Read the model definition and answer for the solid it produces. Units are mm, in the model's axes. A direction names the side the tool comes from. Round coordinates to 2 decimals unless told otherwise and drop trailing zeros. Loops run counter-clockwise (first coordinate to the right, second up) from the corner with the lowest first, then second, coordinate; pieces in that order, holes last. Notation, with made-up numbers: M 9,74 L 37,74 A32 cw 37,100 Z; hole C -12,-2.75 d8. An arc over 180 degrees is marked long. Write each question's results on one line, items separated by ' | '.
Autodesk Inventor part; units mm, degrees
ref_plane "YZ Plane" through (0, 0, 0) normal (1, 0, 0) x (0, 1, 0)
ref_plane "XZ Plane" through (0, 0, 0) normal (0, 1, 0) x (-1, 0, 0)
ref_plane "XY Plane" through (0, 0, 0) normal (0, 0, 1) x (1, 0, 0)
sketch "Szkic1" plane through (0, 0, 0) normal (0, 0, 1) x (1, 0, 0)
  line L0 (-30, -30) -> (30, -30)
  line L1 (30, -30) -> (30, 30)
  line L2 (30, 30) -> (-30, 30)
  line L3 (-30, 30) -> (-30, -30)
  line L4 (-30, -30) -> (30, 30) construction
  line L5 (30, -30) -> (-30, 30) construction
  point P0 (0, 0)
  dimension "d0" = 60
  dimension "d1" = 60
extrude "Wyciągnięcie proste1" add sketch "Szkic1" along normal blind 35
sketch "Szkic2" plane through (0, 0, 35) normal (0, 0, 1) x (1, 0, 0)
  circle A0 centre (0, 0) radius 25
  dimension "d4" = 50
extrude "Wyciągnięcie proste2" cut sketch "Szkic2" against normal blind 12
sketch "Szkic3" plane through (0, 0, 23) normal (0, 0, 1) x (1, 0, 0)
  circle A0 centre (0, 0) radius 14
  dimension "d7" = 28
extrude "Wyciągnięcie proste3" cut sketch "Szkic3" against normal up to next
sketch "Szkic4" plane through (0, 0, 23) normal (0, 0, 1) x (1, 0, 0)
  circle A0 centre (0, 0) radius 19
  circle A1 centre (0, 19) radius 3
  circle A2 centre (-16.4545, 9.5) radius 3
  circle A3 centre (-16.4545, -9.5) radius 3
  circle A4 centre (0, -19) radius 3
  circle A5 centre (16.4545, -9.5) radius 3
  circle A6 centre (16.4545, 9.5) radius 3
  dimension "d10" = 38
  dimension "d11" = 6
  dimension "d14" = 360
sketch "Szkic13" plane through (0, 0, 35) normal (0, 0, 1) x (1, 0, 0)
  circle A0 centre (0, 0) radius 25
  line L0 (-30, -30) -> (30, -30)
  line L1 (30, -30) -> (30, 30)
  line L2 (30, 30) -> (-30, 30)
  line L3 (-30, 30) -> (-30, -30)
extrude "Wyciągnięcie proste10" cut sketch "Szkic13" against normal up to surface (12 mm away)
extrude "Wyciągnięcie proste11" cut sketch "Szkic4" against normal up to next contours A6 A0 | A0 A6 | A5 A0 | A0 A5 | A1 A0 | A0 A1 | A4 A0 | A0 A4 | A2 A0 | A0 A2 | A3 A0 | A0 A3
thread "Gwint7"
thread "Gwint8"
thread "Gwint9"
thread "Gwint10"
thread "Gwint11"
thread "Gwint12"
sketch "Szkic14" plane through (0, 0, 0) normal (0, 0, -1) x (-1, 0, 0)
  circle A0 centre (0, 0) radius 14
  line L0 (30, -30) -> (-30, -30)
  line L1 (30, 30) -> (30, -30)
  line L2 (-30, 30) -> (30, 30)
  line L3 (-30, -30) -> (-30, 30)
extrude "Wyciągnięcie proste12" cut sketch "Szkic14" against normal blind 3
sketch "Szkic16" plane through (-30, -30, 23) normal (0, -1, 0) x (1, 0, 0)
  line L0 (0, -20) -> (60, -20)
  line L1 (60, -20) -> (60, 0)
  line L2 (60, 0) -> (0, 0)
  line L3 (0, -20) -> (0, 0)
  point P0 (30, -23)
extrude "Wyciągnięcie proste14" add sketch "Szkic16" along normal blind 20
sketch "Szkic17" plane through (0, 0, 23) normal (0, 0, 1) x (1, 0, 0)
  circle A0 centre (16.4545, 9.5) radius 3
  circle A1 centre (0, -19) radius 3
  circle A2 centre (-16.4545, 9.5) radius 3
  circle A3 centre (0, 19) radius 3
  circle A4 centre (-16.4545, -9.5) radius 3
  circle A5 centre (16.4545, -9.5) radius 3
  line L0 (30, 30) -> (30, -50)
  line L1 (-30, 30) -> (30, 30)
  line L2 (-30, -50) -> (-30, 30)
  line L3 (30, -50) -> (-30, -50)
  circle A6 centre (0, 0) radius 14
  line L4 (-30, -50) -> (-30, -40)
  line L5 (-30, 30) -> (-30, -50)
  line L6 (-30, -40) -> (30, -40)
  line L7 (30, -50) -> (30, 30)
  line L8 (-30, -40) -> (-18, -40)
  line L9 (-18, -40) -> (-6, -40)
  line L10 (-6, -40) -> (6, -40)
  line L11 (6, -40) -> (18, -40)
  circle A7 centre (-18, -40) radius 2.5
  circle A8 centre (-6, -40) radius 2.5
  circle A9 centre (6, -40) radius 2.5
  circle A10 centre (18, -40) radius 2.5
  dimension "d100" = 10
  dimension "d101" = 12
  dimension "d102" = 12
  dimension "d103" = 12
  dimension "d104" = 12
  dimension "d105" = 5
  dimension "d106" = 5
  dimension "d107" = 5
  dimension "d108" = 5
hole "Otwór1" at (-18, -40, 23) at (-6, -40, 23) at (6, -40, 23) at (18, -40, 23) direction (0, 0, -1) diameter 5 end through all counterbore diameter 9 counterbore depth 5
properties part number "Obudowa nakrętki trapezowej fi 16 - oś Y"
1. Find section B-B, the plane z = 6. Count the separate pieces of the cut face and the enclosed holes in it, then the cut area to 3 significant figures.
Completed:
separate pieces: 1 | enclosed holes: 11 | area: 3,940 mm2
2. Find section A-A, the plane y = 0. Give the vertices of the cut face in (x, z), then the cut area to 3 significant figures.
Completed:
outline: M -30,3 L -14,3 L -14,23 L -30,23 Z; M 14,3 L 30,3 L 30,23 L 14,23 Z | area: 640 mm2
3. Given P1, Ø4, axis at x = -6, y = -40, coming from the +Z side; P2, Ø4.5, axis at x = -7, y = -39, coming from the +Z side, each flat-ended and moving along its own axis, determine where each tip first touches the part or whether it passes through.
Completed:
P1: passes through | P2: stops at z = 18
4. Find section D-D, the plane y = 9.5. Give the vertices of the cut face in (x, z), then the cut area to 3 significant figures.
Completed:
outline: M -30,3 L -19.45,3 L -19.45,23 L -30,23 Z; M -13.45,3 L -10.28,3 L -10.28,23 L -13.45,23 Z; M 10.28,3 L 13.45,3 L 13.45,23 L 10.28,23 Z; M 19.45,3 L 30,3 L 30,23 L 19.45,23 Z | area: 549 mm2
5. Determine the mould class of faces 1 (the face through (-30, -9, 13)), 2 (the face through (19.226, 8.351, 13.14)), 3 (the face through (0, -50, 13)) for opening direction Y: released by +Y, released by -Y, zero draft, split by the parting line, or undercut.
Completed:
face 1: zero draft | face 2: undercut | face 3: released by -Y
6. Find section C-C, the plane x = -6. Give the vertices of the cut face in (y, z).
Completed:
outline: M -50,3 L -42.5,3 L -42.5,18 L -44.5,18 L -44.5,23 L -50,23 Z; M -37.5,3 L -12.65,3 L -12.65,23 L -35.5,23 L -35.5,18 L -37.5,18 Z; M 12.65,3 L 30,3 L 30,23 L 12.65,23 Z
7. Which of the six approach directions +Z, -Z, +X, -X, +Y, -Y give full straight-line access (tool end or side, diameter ignored) to faces 4 (the face through (-19.45, 9.63, 13.14)), 5 (the face through (-7.352, -44.292, 20.465))?
Completed:
face 4: +Z, -Z | face 5: +Z
8. Find the intervals of material crossed by L1, parallel to X at y = -40, z = 22; L2, parallel to X at y = 19, z = 18.5; L3, parallel to X at y = -40, z = 7.25, in increasing order.
Completed:
L1: x = -30 to -22.5, -13.5 to -10.5, -1.5 to 1.5, 10.5 to 13.5, 22.5 to 30 | L2: x = -30 to -3, 3 to 30 | L3: x = -30 to -20.5, -15.5 to -8.5, -3.5 to 3.5, 8.5 to 15.5, 20.5 to 30
